```python
from build123d import *

# Parameters (mm, degrees)
SKETCH_R        = 80
PAD_DEPTH       = 5
PAD001_DEPTH    = 40
SKETCH003_W     = 90
SKETCH003_H     = 90
POCKET_DEPTH    = 40
SKETCH004_R     = 1.75
POCKET001_DEPTH = 45.001
SKETCH005_R     = 17
SKETCH005_R_2   = 60
POCKET002_DEPTH = 5.001
SKETCH006_R     = 16
POCKET003_DEPTH = 119.674913
SKETCH007_R     = 16
POCKET004_DEPTH = 119.674913
PAD002_DEPTH    = 10
SKETCH010_R     = 1.75
POCKET005_DEPTH = 119.674913


with BuildPart() as part:
    # Sketch → Pad (new body)
    with BuildSketch(Plane.XY):
        Circle(SKETCH_R)
    extrude(amount=PAD_DEPTH)

    # Sketch002 → Pad001 (new body)
    with BuildSketch(Plane.XY.offset(5)):
        with BuildLine():
            ThreePointArc((-47.145878, 50), (-55.712311, 55.712311), (-50, 47.145878))
            Line((-50, -47.145878), (-50, 47.145878))
            ThreePointArc((-50, -47.145878), (-55.712311, -55.712311), (-47.145878, -50))
            Line((47.145878, -50), (-47.145878, -50))
            ThreePointArc((47.145878, -50), (55.712311, -55.712311), (50, -47.145878))
            Line((50, 47.145878), (50, -47.145878))
            ThreePointArc((50, 47.145878), (55.712311, 55.712311), (47.145878, 50))
            Line((-47.145878, 50), (47.145878, 50))
        make_face()
    extrude(amount=PAD001_DEPTH)

    # Sketch003 → Pocket (cut)
    with BuildSketch(Plane.XY.offset(45)):
        Rectangle(SKETCH003_W, SKETCH003_H)
    extrude(amount=-POCKET_DEPTH, mode=Mode.SUBTRACT)

    # Sketch004 → Pocket001 (cut, through all)
    with BuildSketch(Plane.XY.offset(45)):
        with Locations((-52, -52)):
            Circle(SKETCH004_R)
        with Locations((52, 52)):
            Circle(SKETCH004_R)
        with Locations((52, -52)):
            Circle(SKETCH004_R)
        with Locations((-52, 52)):
            Circle(SKETCH004_R)
    extrude(amount=-POCKET001_DEPTH, mode=Mode.SUBTRACT)

    # Sketch005 → Pocket002 (cut, through all)
    with BuildSketch(Plane.XY.offset(5)):
        with Locations((-22.5, 22.5)):
            Circle(SKETCH005_R)
        with Locations((22.5, 22.5)):
            Circle(SKETCH005_R)
        with Locations((-22.5, -22.5)):
            Circle(SKETCH005_R)
        with Locations((22.5, -22.5)):
            Circle(SKETCH005_R)
        with Locations((0, -115)):
            Circle(SKETCH005_R_2)
        with Locations((-115, 0)):
            Circle(SKETCH005_R_2)
        with Locations((115, 0)):
            Circle(SKETCH005_R_2)
        with Locations((0, 115)):
            Circle(SKETCH005_R_2)
    extrude(amount=-POCKET002_DEPTH, mode=Mode.SUBTRACT)

    # Sketch006 → Pocket003 (cut, through all)
    with BuildSketch(Plane.YZ.offset(50)):
        with Locations((0, 25)):
            Circle(SKETCH006_R)
        with BuildLine():
            ThreePointArc((-32.145878, 50), (-37.145878, 45), (-32.145878, 40))
            Line((-32.145878, 40), (-22.145878, 40))
            ThreePointArc((-22.145878, 40), (-17.145878, 45), (-22.145878, 50))
            Line((-32.145878, 50), (-22.145878, 50))
        make_face()
        with BuildLine():
            ThreePointArc((22.145904, 50), (17.145878, 45.000013), (22.145878, 40))
            Line((22.145878, 40), (32.145878, 40))
            ThreePointArc((32.145878, 40), (37.145878, 44.999989), (32.1459, 50))
            Line((22.145904, 50), (32.1459, 50))
        make_face()
        with BuildLine():
            ThreePointArc((-32.145847, 20), (-37.145878, 15.000015), (-32.145878, 10))
            Line((-32.145878, 10), (-22.145878, 10))
            ThreePointArc((-22.145878, 10), (-17.145878, 14.999986), (-22.145849, 20))
            Line((-32.145847, 20), (-22.145849, 20))
        make_face()
        with BuildLine():
            ThreePointArc((22.145861, 20), (17.145878, 14.999992), (22.145878, 10))
            Line((22.145878, 10), (32.145878, 10))
            ThreePointArc((32.145878, 10), (37.145878, 15.000009), (32.14586, 20))
            Line((22.145861, 20), (32.14586, 20))
        make_face()
    extrude(amount=-POCKET003_DEPTH, mode=Mode.SUBTRACT)

    # Sketch007 → Pocket004 (cut, through all)
    with BuildSketch(Plane.XZ.offset(50)):
        with Locations((0, 25)):
            Circle(SKETCH007_R)
        with BuildLine():
            ThreePointArc((-32.145883, 50), (-37.145878, 45), (-32.145883, 40))
            Line((-32.145883, 40), (-22.145873, 40))
            ThreePointArc((-22.145873, 40), (-17.145878, 45), (-22.145873, 50))
            Line((-32.145883, 50), (-22.145873, 50))
        make_face()
        with BuildLine():
            ThreePointArc((32.145897, 40), (37.145878, 45), (32.145898, 50))
            Line((32.145898, 50), (22.145895, 50))
            ThreePointArc((22.145895, 50), (17.145878, 45.000001), (22.145893, 40))
            Line((32.145897, 40), (22.145893, 40))
        make_face()
        with BuildLine():
            ThreePointArc((-32.145897, 20), (-37.145878, 14.99999), (-32.145878, 10))
            Line((-32.145878, 10), (-22.145878, 10))
            ThreePointArc((-22.145878, 10), (-17.145878, 15.000011), (-22.145899, 20))
            Line((-32.145897, 20), (-22.145899, 20))
        make_face()
        with BuildLine():
            ThreePointArc((22.145901, 20), (17.145878, 15.000011), (22.145878, 10))
            Line((22.145878, 10), (32.145878, 10))
            ThreePointArc((32.145878, 10), (37.145878, 14.999989), (32.1459, 20))
            Line((22.145901, 20), (32.1459, 20))
        make_face()
    extrude(amount=-POCKET004_DEPTH, mode=Mode.SUBTRACT)

    # Sketch008 → Pad002 (new body)
    with BuildSketch(Plane(origin=(0, 0, 0), x_dir=(1, 0, 0), z_dir=(0, 0, -1))):
        with BuildLine():
            ThreePointArc((-40.000017, 53), (-45, 48), (-40.000017, 43))
            Line((-40.000017, 43), (39.999994, 43))
            ThreePointArc((39.999994, 43), (45, 48), (39.999994, 53))
            Line((-40.000017, 53), (39.999994, 53))
        make_face()
        with BuildLine():
            ThreePointArc((-39.99998, -43), (-45, -48), (-39.99998, -53))
            Line((-39.99998, -53), (40.00001, -53))
            ThreePointArc((40.00001, -53), (45, -48), (40.00001, -43))
            Line((-39.99998, -43), (40.00001, -43))
        make_face()
    extrude(amount=PAD002_DEPTH)

    # Sketch010 → Pocket005 (cut, through all)
    with BuildSketch(Plane(origin=(0, 50, 0), x_dir=(-1, 0, 0), z_dir=(0, 1, 0))):
        with Locations((-40, 34.992924)):
            Circle(SKETCH010_R)
        with Locations((-40, 10)):
            Circle(SKETCH010_R)
        with Locations((40, 10)):
            Circle(SKETCH010_R)
        with Locations((40, 34.941413)):
            Circle(SKETCH010_R)
    extrude(amount=-POCKET005_DEPTH, mode=Mode.SUBTRACT)


solid = part.part
```
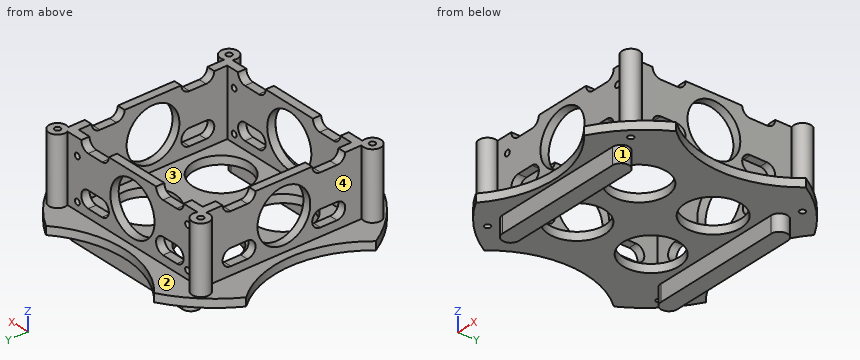
Work out the finished part from the listing and answer in its coordinate system (mm). Face numbers are marked on the shaded views. A direction names the side the tool comes from. Give positions to 0.01 mm unless a question says otherwise; leave off trailing zeros. Loops run counter-clockwise (first coordinate to the right, second up) from the corner with the lowest first, then second, coordinate; pieces in that order, holes last. Notation, with made-up numbers: (8.25, 24) -> (38.25, 24) arc R24 ccw to (38.25, 51) -> close; hole circle Ø5 at (-8, 24.25). An arc over 180 degrees is marked (long way). Put each result on its own line as item: value. Start each with the question number.
Item 1: The mould has two halves that part along Y. Classify the marked faces 3 and 4: released by +Y, released by -Y, zero draft, split by the parting line, or undercut.
Item 2: The part is cut by section D-D (z = 15). State how many separate pieces and enclosed holes the cut face has, then the cut area to 3 significant figures.
Item 3: Each of these flat-tipped pins is pushed along its axis until it touches: P1, Ø4.5, axis at x = 40, z = 10, coming from the +Y side; P2, Ø1.5, axis at x = 48, y = 27, coming from the +Z side; P3, Ø20.5, axis at x = -22.5, y = 22.5, coming from the -Z side; P4, Ø8, axis at y = -46.5, z = 1, coming from the -X side. Where does it stop, or does it pass through?
Item 4: Find the intervals of material crossed by L1, parallel to Y at x = 52, z = 20; L2, parallel to Z at x = 40, y = -46.25; L3, parallel to Y at x = 49.5, z = 12, in increasing order. Write a range as [from, to].
Item 5: The part is cut by section A-A (x = 0). Give the vertices of the cut face in (y, z).
Item 6: The part is cut by section C-C (y = 60.5). Give the vertices of the cut face in (x, z).
Item 7: Which of the six approach directions +Z, -Z, +X, -X, +Y, -Y give full straight-line access (tool end or side, diameter ignored) to the marked faces 1 and 2?
Item 8: The part is cut by section B-B (y = 0). Give the vertices of the cut face in (x, z), then the cut area to 3 significant figures.
Answers below:
1. face 3: undercut
1. face 4: undercut
2. separate pieces: 12
2. enclosed holes: 4
2. area: 888 mm2
3. P1: y = 50
3. P2: z = 40
3. P3: through
3. P4: x = -67.78
4. L1: [-57.25, -53.75], [-50.25, -46.75], [46.75, 50.25], [53.75, 57.25]
4. L2: [-10, 8.25], [11.75, 33.24], [36.74, 45]
4. L3: [-56.62, -36.15], [-18.15, -9.33], [9.33, 18.15], [36.15, 56.62]
5. outline: (-55, 0) -> (-53, 0) -> (-53, -10) -> (-43, -10) -> (-43, 0) -> (43, 0) -> (43, -10) -> (53, -10) -> (53, 0) -> (55, 0) -> (55, 5) -> (50, 5) -> (50, 9) -> (45, 9) -> (45, 5) -> (-45, 5) -> (-45, 9) -> (-50, 9) -> (-50, 5) -> (-55, 5) -> close; (-50, 41) -> (-45, 41) -> (-45, 45) -> (-50, 45) -> close; (45, 41) -> (50, 41) -> (50, 45) -> (45, 45) -> close
6. outline: (-52.34, 0) -> (-25.09, 0) -> (-25.09, 5) -> (-52.34, 5) -> close; (25.09, 0) -> (52.34, 0) -> (52.34, 5) -> (25.09, 5) -> close
7. face 1: -Z, +X
7. face 2: +Z
8. outline: (-55, 0) -> (55, 0) -> (55, 5) -> (50, 5) -> (50, 9) -> (45, 9) -> (45, 5) -> (-45, 5) -> (-45, 9) -> (-50, 9) -> (-50, 5) -> (-55, 5) -> close; (-50, 41) -> (-45, 41) -> (-45, 45) -> (-50, 45) -> close; (45, 41) -> (50, 41) -> (50, 45) -> (45, 45) -> close
8. area: 630 mm2
